Answer from the drawing. Dimensions are ordinates in mm from the lowest x, y and z of the part. A direction names the side the tool comes from. Round coordinates to 2 decimals unless told otherwise and drop trailing zeros. Order: outer loops, then holes, each group sorted by start corner. A loop starts at its lowest first (then second) coordinate and runs counter-clockwise, first axis right, second up. Notation, with made-up numbers: M 56.5,35.5 L 89.5,35.5 A13 ccw 89.5,42.5 Z; hole C -37,73 d8. An arc over 180 degrees is marked long. Write item = value, one per line. Start each with the question number.
(1) Each of these flat-tipped pins is pushed along its axis until it touches: pin 1 (6 mm diameter, centred on x = 19, z = 1.5, fed in from -Y); pin 2 (5 mm diameter, centred on y = 7, z = 8, fed in from -X); pin 3 (6 mm diameter, centred on x = 18.5, z = 8.5, fed in from +Y). Where does it stop, or does it pass through?
(2) A cutting plane is placed at A-A, the plane x = 11. Determine the outline of the cut face in (y, z), and give its area (3 significant figures).
(3) A cutting plane is placed at D-D, the plane z = 8.5. Determine the outline of the cut face in (x, y).
(4) Straight lines are drawn through the part: probe 1 along Y at (x, z) = (11, 1); probe 2 along Y at (x, z) = (11, 8.25); probe 3 along Z at (x, y) = (6.25, 18). For each, find the intervals that lie inside material, in ascending order. Write a range as from..to.
(5) For a pull along X with two mould halves and no side action, classify the marked faces 1, 2 and 3 as released by +X, released by -X, zero draft, split by the parting line, or undercut.
(6) Which of the six approach directions +Z, -Z, +X, -X, +Y, -Y give full straight-line access (tool end or side, diameter ignored) to the marked faces 4 and 5?
(7) A cutting plane is placed at C-C, the plane x = 18.25. Determine the outline of the cut face in (y, z), and give its area (3 significant figures).
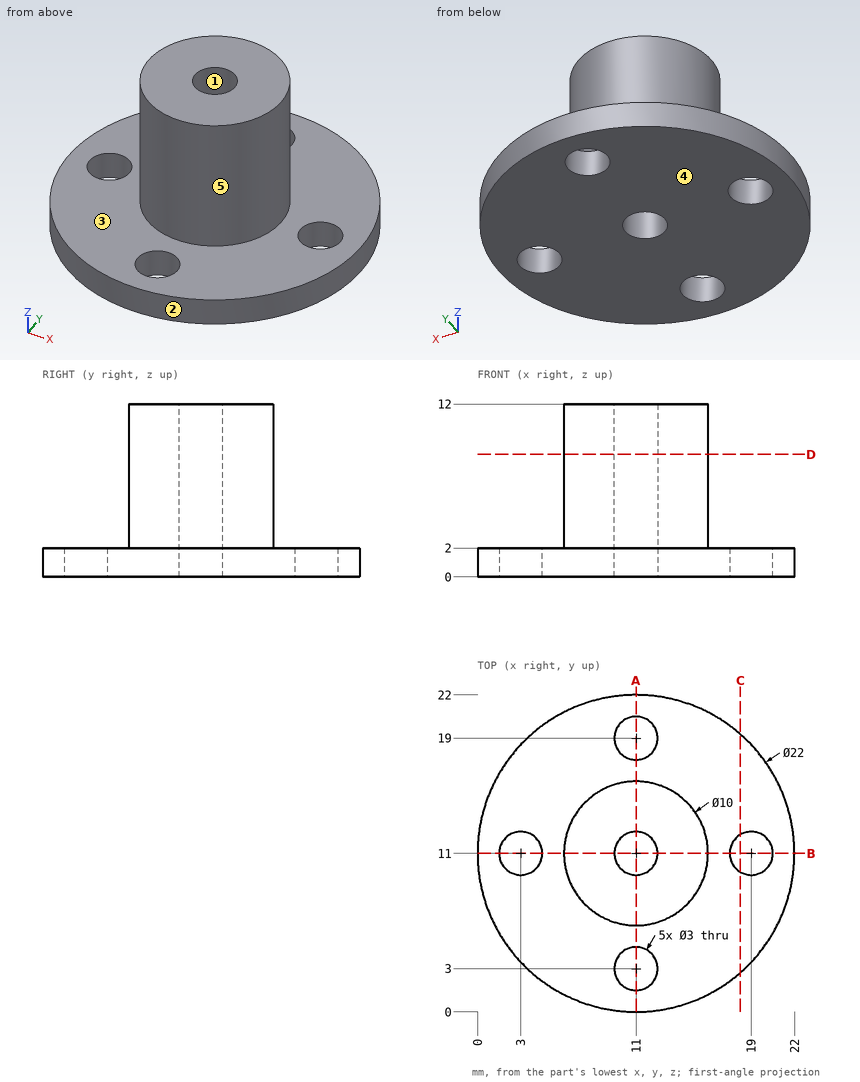
Reported:
q1.pin_1 = 1.2
q1.pin_2 = 6.23
q1.pin_3 = 13.18
q2.outline = M 0,0 L 1.5,0 L 1.5,2 L 0,2 Z; M 4.5,0 L 9.5,0 L 9.5,12 L 6,12 L 6,2 L 4.5,2 Z; M 12.5,0 L 17.5,0 L 17.5,2 L 16,2 L 16,12 L 12.5,12 Z; M 20.5,0 L 22,0 L 22,2 L 20.5,2 Z
q2.area = 96.0 mm²
q3.outline = C 11,11 d10; hole C 11,11 d3
q4.probe_1 = 0..1.5, 4.5..9.5, 12.5..17.5, 20.5..22
q4.probe_2 = 6..9.5, 12.5..16
q4.probe_3 = 0..2
q5.face_1 = undercut
q5.face_2 = split by the parting line
q5.face_3 = zero draft
q6.face_4 = -Z, +X, -X, +Y, -Y
q6.face_5 = +Z
q7.outline = M 2.73,0 L 9.7,0 L 9.7,2 L 2.73,2 Z; M 12.3,0 L 19.27,0 L 19.27,2 L 12.3,2 Z
q7.area = 27.9 mm²
